Geometry check sheet. Reference: the model listing, model coordinates, mm. Face numbers are marked on the shaded views. A direction names the side the tool comes from. Coordinates: 2 decimals unless noted, no trailing zeros. Loops run counter-clockwise (first coordinate to the right, second up) from the corner with the lowest first, then second, coordinate; pieces in that order, holes last. Notation, with made-up numbers: M -7,-7 L 47,-7 A30 cw 47,31 Z; hole C 39,53 d2. An arc over 180 degrees is marked long. One line per question, with ' | ' between items. Start each with the question number.
from build123d import *

# Parameters (mm, degrees)
SKETCH1_W           = 6.92
SKETCH1_H           = 12
BOSS_EXTRUDE1_DEPTH = 0.53
SKETCH2_W           = 5
SKETCH2_H           = 5
BOSS_EXTRUDE2_DEPTH = 1.57
SKETCH3_R           = 2
CUT_EXTRUDE1_DEPTH  = 0.2
CHAMFER1_SIZE       = 0.1
SKETCH6_W           = 2
SKETCH6_H           = 1.2
BOSS_EXTRUDE3_DEPTH = 0.45
CUT_EXTRUDE2_DEPTH  = 0.1


with BuildPart() as part:
    # Sketch1 → Boss-Extrude1 (new body)
    with BuildSketch(Plane(origin=(0, 0, 0), x_dir=(1, 0, 0), z_dir=(0, 1, 0))):
        Rectangle(SKETCH1_W, SKETCH1_H)
    extrude(amount=BOSS_EXTRUDE1_DEPTH)

    # Sketch2 → Boss-Extrude2 (add)
    with BuildSketch(Plane.XZ):
        Rectangle(SKETCH2_W, SKETCH2_H)
    extrude(amount=BOSS_EXTRUDE2_DEPTH)

    # Sketch3 → Cut-Extrude1 (cut)
    with BuildSketch(Plane.XZ.offset(1.57)):
        with Locations(Location((0, 0, 0), (0, 0, 270))):
            Circle(SKETCH3_R)
    extrude(amount=-CUT_EXTRUDE1_DEPTH, mode=Mode.SUBTRACT)

    # Chamfer1
    chamfer1_edges = [part.edges().sort_by_distance(p)[0] for p in [
        (0, -1.57, 2),
    ]]
    chamfer(chamfer1_edges, length=CHAMFER1_SIZE)

    # Sketch6 → Boss-Extrude3 (add)
    with BuildSketch(Plane.XZ):
        with Locations((0, -4.25)):
            Rectangle(SKETCH6_W, SKETCH6_H)
    extrude(amount=BOSS_EXTRUDE3_DEPTH)

    # Sketch4 → Cut-Extrude2 (cut)
    with BuildSketch(Plane.XZ):
        with BuildLine():
            Line((3.46, 0.85), (3.46, -0.85))
            ThreePointArc((3.46, -0.85), (2.61, 0), (3.46, 0.85))
        make_face()
        with BuildLine():
            Line((3.46, 5.151541621), (2.351035145, 5.151541621))
            ThreePointArc((2.351035145, 5.151541621), (1.501035145, 4.301541621), (2.351035145, 3.451541621))
            Line((2.351035145, 3.451541621), (3.46, 3.451541621))
            Line((3.46, 3.451541621), (3.46, 5.151541621))
        make_face()
        with BuildLine():
            Line((3.46, -5.151541621), (2.351035145, -5.151541621))
            ThreePointArc((2.351035145, -5.151541621), (1.501035145, -4.301541621), (2.351035145, -3.451541621))
            Line((2.351035145, -3.451541621), (3.46, -3.451541621))
            Line((3.46, -3.451541621), (3.46, -5.151541621))
        make_face()
        with BuildLine():
            Line((-2.351035145, -3.451541621), (-3.46, -3.451541621))
            Line((-3.46, -3.451541621), (-3.46, -5.151541621))
            Line((-3.46, -5.151541621), (-2.351035145, -5.151541621))
            ThreePointArc((-2.351035145, -5.151541621), (-1.501035145, -4.301541621), (-2.351035145, -3.451541621))
        make_face()
        with BuildLine():
            Line((-3.46, 3.451541621), (-3.46, 5.151541621))
            Line((-3.46, 5.151541621), (-2.351035145, 5.151541621))
            ThreePointArc((-2.351035145, 5.151541621), (-1.501035145, 4.301541621), (-2.351035145, 3.451541621))
            Line((-2.351035145, 3.451541621), (-3.46, 3.451541621))
        make_face()
        with BuildLine():
            Line((-3.46, 0.85), (-3.46, -0.85))
            ThreePointArc((-3.46, -0.85), (-2.61, 0), (-3.46, 0.85))
        make_face()
    extrude(amount=-CUT_EXTRUDE2_DEPTH, mode=Mode.SUBTRACT)


solid = part.part
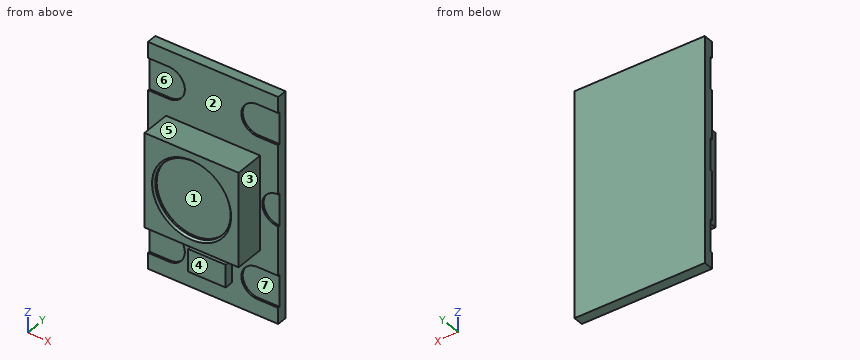
1. Tool access check on the marked faces 4, 5, 6 and 7. Record the directions out of +Z, -Z, +X, -X, +Y, -Y that give a thin tool (end or side, any length) a straight path to the whole face; none if there is none.
2. Depth check by flat-ended pin: pin 1 Ø1.9 at (x, z) = (3, 4.5) entering from -Y; pin 2 Ø1.3 at (x, z) = (0, -4) entering from -Y; pin 3 Ø3 at (x, z) = (-2, -3) entering from -Y; pin 4 Ø0.8 at (x, z) = (2.5, -4) entering from -Y. Enter the tip coordinate at first touch or a pass-through.
3. Sectioned sample at B-B (y = -0.6). Record the cut outline in (x, z), and give its area (3 significant figures).
4. Sectioned sample at C-C (z = 3). Record the cut outline in (x, y).
5. Draft check along X on the marked faces 1, 2 and 3. Enter one of: +X half, -X half, draft (parallel to the pull), parting line (faces both ways), or undercut.
6. Sectioned sample at A-A (z = 0). Record the cut outline in (x, y), and give its area (3 significant figures).
7. Thickness scan on line 1 (Z direction, x = -1.5, y = -0.5); line 2 (Y direction, x = -1, z = 3); line 3 (Y direction, x = -2, z = 4.5). Record the ranges inside material, lowest first.
Result:
1) face 4: -Z, +X, -X, -Y | face 5: +Z, +X, -X, -Y | face 6: -X, -Y | face 7: +X, -Y
2) pin 1: stops at y = 0 | pin 2: stops at y = -0.45 | pin 3: stops at y = -1.57 | pin 4: stops at y = 0.1
3) outline: M -2.5,-2.5 L 2.5,-2.5 L 2.5,2.5 L -2.5,2.5 Z | area: 25.0 mm2
4) outline: M -3.46,0 L 3.46,0 L 3.46,0.53 L -3.46,0.53 Z
5) face 1: undercut | face 2: draft | face 3: +X half
6) outline: M -3.46,0.1 L -2.61,0.1 L -2.61,0 L -2.5,0 L -2.5,-1.57 L -2.1,-1.57 L -2,-1.47 L -2,-1.37 L 2,-1.37 L 2,-1.47 L 2.1,-1.57 L 2.5,-1.57 L 2.5,0 L 2.61,0 L 2.61,0.1 L 3.46,0.1 L 3.46,0.53 L -3.46,0.53 Z | area: 10.5 mm2
7) line 1: z = -2.5 to 2.5 | line 2: y = 0 to 0.53 | line 3: y = 0.1 to 0.53
